CAD build for the part. Positions are in the model's coordinates, mm. Round coordinates to 2 decimals unless told otherwise and drop trailing zeros. Order: outer loops, then holes, each group sorted by start corner. A loop starts at its lowest first (then second) coordinate and runs counter-clockwise, first axis right, second up. Notation, with made-up numbers: M -8,-21 L 20,-21 A20 ccw 20,14 Z; hole C 43,80.5 d11. An arc over 180 degrees is marked long. Put each result on its own line as item: value.
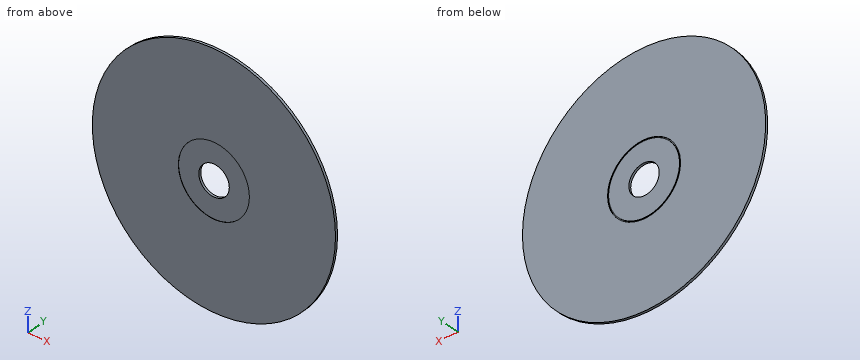
```python
from build123d import *

# Parameters (mm, degrees)
SKETCH1_R           = 60
SKETCH1_R_2         = 7.5
BOSS_EXTRUDE1_DEPTH = 1.2
SKETCH2_R           = 18
SKETCH2_R_2         = 17.5
CUT_EXTRUDE1_DEPTH  = 0.3
SKETCH4_R           = 17.5
CUT_EXTRUDE2_DEPTH  = 0.1


with BuildPart() as part:
    # Sketch1 → Boss-Extrude1 (new body)
    with BuildSketch(Plane(origin=(0, 0, 0), x_dir=(1, 0, 0), z_dir=(0, 1, 0))):
        Circle(SKETCH1_R)
        Circle(SKETCH1_R_2, mode=Mode.SUBTRACT)
    extrude(amount=BOSS_EXTRUDE1_DEPTH)

    # Sketch2 → Cut-Extrude1 (cut)
    with BuildSketch(Plane(origin=(0, 1.2, 0), x_dir=(1, 0, 0), z_dir=(0, 1, 0))):
        Circle(SKETCH2_R)
        Circle(SKETCH2_R_2, mode=Mode.SUBTRACT)
    extrude(amount=-CUT_EXTRUDE1_DEPTH, mode=Mode.SUBTRACT)

    # Sketch4 → Cut-Extrude2 (cut)
    with BuildSketch(Plane.XZ):
        Circle(SKETCH4_R)
    extrude(amount=-CUT_EXTRUDE2_DEPTH, mode=Mode.SUBTRACT)


solid = part.part
```
Item 1: Band-saw the part on C-C on y = 0.4. Give the cut face in (x, z).
Answers below:
outline: C 0,0 d120; hole C 0,0 d15
Item 2: Band-saw the part on B-B on x = 0. Give the cut face in (y, z), and give its area (3 significant figures).
Answers below:
outline: M 0,-60 L 1.2,-60 L 1.2,-18 L 0.9,-18 L 0.9,-17.5 L 1.2,-17.5 L 1.2,-7.5 L 0.1,-7.5 L 0.1,-17.5 L 0,-17.5 Z; M 0,17.5 L 0.1,17.5 L 0.1,7.5 L 1.2,7.5 L 1.2,17.5 L 0.9,17.5 L 0.9,18 L 1.2,18 L 1.2,60 L 0,60 Z
area: 124 mm²
Item 3: Band-saw the part on A-A on z = 0. Give the cut face in (x, y).
Answers below:
outline: M -60,0 L -17.5,0 L -17.5,0.1 L -7.5,0.1 L -7.5,1.2 L -17.5,1.2 L -17.5,0.9 L -18,0.9 L -18,1.2 L -60,1.2 Z; M 7.5,0.1 L 17.5,0.1 L 17.5,0 L 60,0 L 60,1.2 L 18,1.2 L 18,0.9 L 17.5,0.9 L 17.5,1.2 L 7.5,1.2 Z
Item 4: Band-saw the part on D-D on z = 46. Give the cut face in (x, y), and give its area (3 significant figures).
Answers below:
outline: M -38.52,0 L 38.52,0 L 38.52,1.2 L -38.52,1.2 Z
area: 92.5 mm²
Item 5: Probe line 1 along X through (y, z) = (1.15, 0); line 2 along X through (y, z) = (0.15, 0). List the from-to ranges inside material, lowest first. Write a range as [from, to].
Answers below:
line 1: [-60, -18], [-17.5, -7.5], [7.5, 17.5], [18, 60]
line 2: [-60, -7.5], [7.5, 60]
